The figure shows three views and two pictorial views of one solid part (mm, origin at its lowest corner). Answer the questions. A direction names the side the tool comes from. Coordinates: 2 decimals unless noted, no trailing zeros. Order: outer loops, then holes, each group sorted by start corner. A loop starts at its lowest first (then second) coordinate and runs counter-clockwise, first axis right, second up. Notation, with made-up numbers: (77, 45.25) - (124, 45.25) arc R22 cw to (124, 74.25) - close; hole circle Ø6 at (78, 61). An arc over 180 degrees is marked (long way). Use one line per item in the form item = value. Start each with the question number.
Item 1: Section A-A, the plane z = 4.15 is taken. Write down the section's boundary in (x, y) (1 decimal), and give its area (3 significant figures).
Item 2: The mould has two halves that part along Z. Classify the marked faces 3, 4 and 5: released by +Z, released by -Z, zero draft, split by the parting line, or undercut.
Item 3: A tool of negligible diameter and unlimited length cuts with its end or side. For the marked faces 1 and 2, from which of +Z, -Z, +X, -X, +Y, -Y can it reach the whole face along a straight path? Write none if from no direction.
Item 4: Consider line 1 along Y through (x, z) = (3.75, 2.25); line 2 along Y through (x, z) = (5, 1.25); line 3 along Z through (x, y) = (4, 19). Determine where each line is inside the solid, lowest interval first. Write a range as [from, to].
Item 5: Each of these flat-tipped pins is pushed along its axis until it touches: pin 1 Ø3 at (y, z) = (1, 4) entering from -X; pin 2 Ø4 at (y, z) = (22, 5) entering from -X (3 decimals); pin 3 Ø1.4 at (x, z) = (4.5, 4) entering from -Y; pin 4 Ø4 at (x, y) = (2.5, 29) entering from +Z (3 decimals). Where does it stop, or does it pass through?
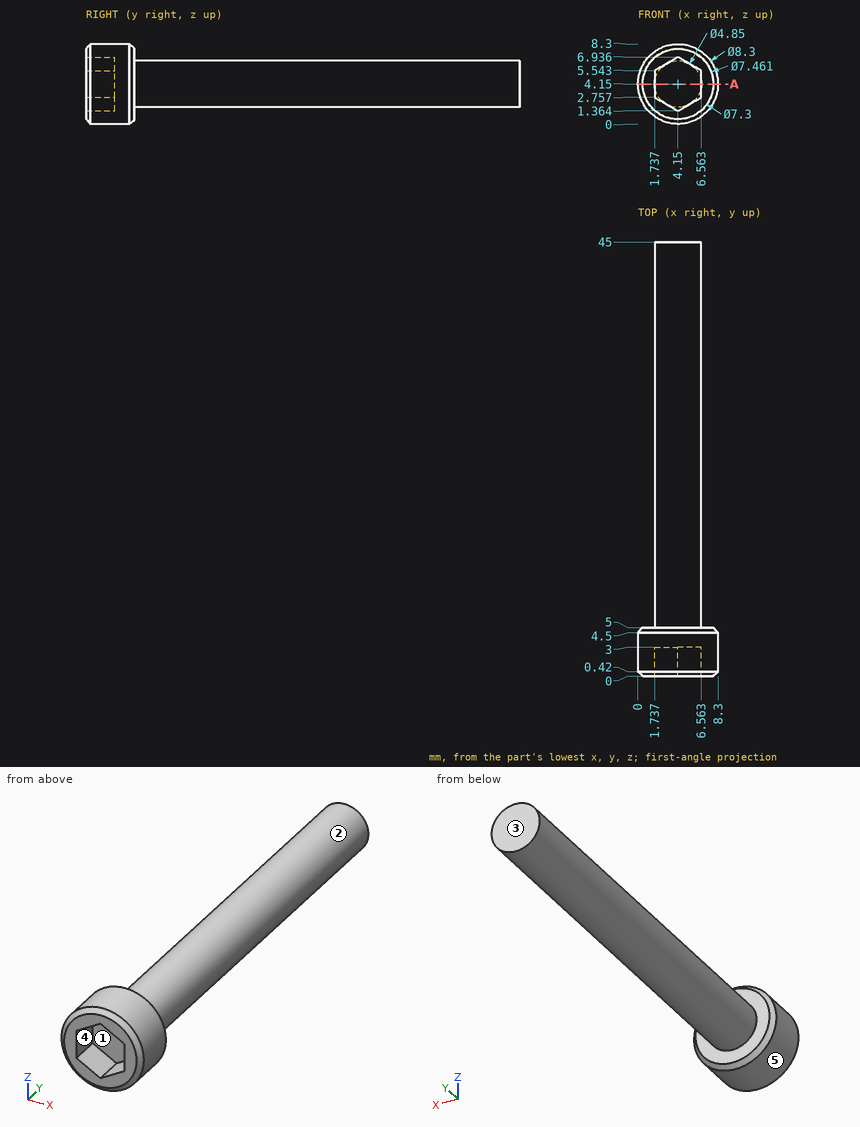
Response:
q1.outline = (0, 0.4) - (0.5, 0) - (1.7, 0) - (1.7, 3) - (6.6, 3) - (6.6, 0) - (7.8, 0) - (8.3, 0.4) - (8.3, 4.5) - (7.9, 5) - (6.6, 5) - (6.6, 45) - (1.7, 45) - (1.7, 5) - (0.4, 5) - (0, 4.5) - close
q1.area = 221 mm2
q2.face_3 = zero draft
q2.face_4 = undercut
q2.face_5 = split by the parting line
q3.face_1 = -Y
q3.face_2 = +Y
q4.line_1 = [3, 45]
q4.line_2 = [0, 5]
q4.line_3 = [1.73, 6.57]
q5.pin_1 = 0
q5.pin_2 = 1.725
q5.pin_3 = 3
q5.pin_4 = 6.575
